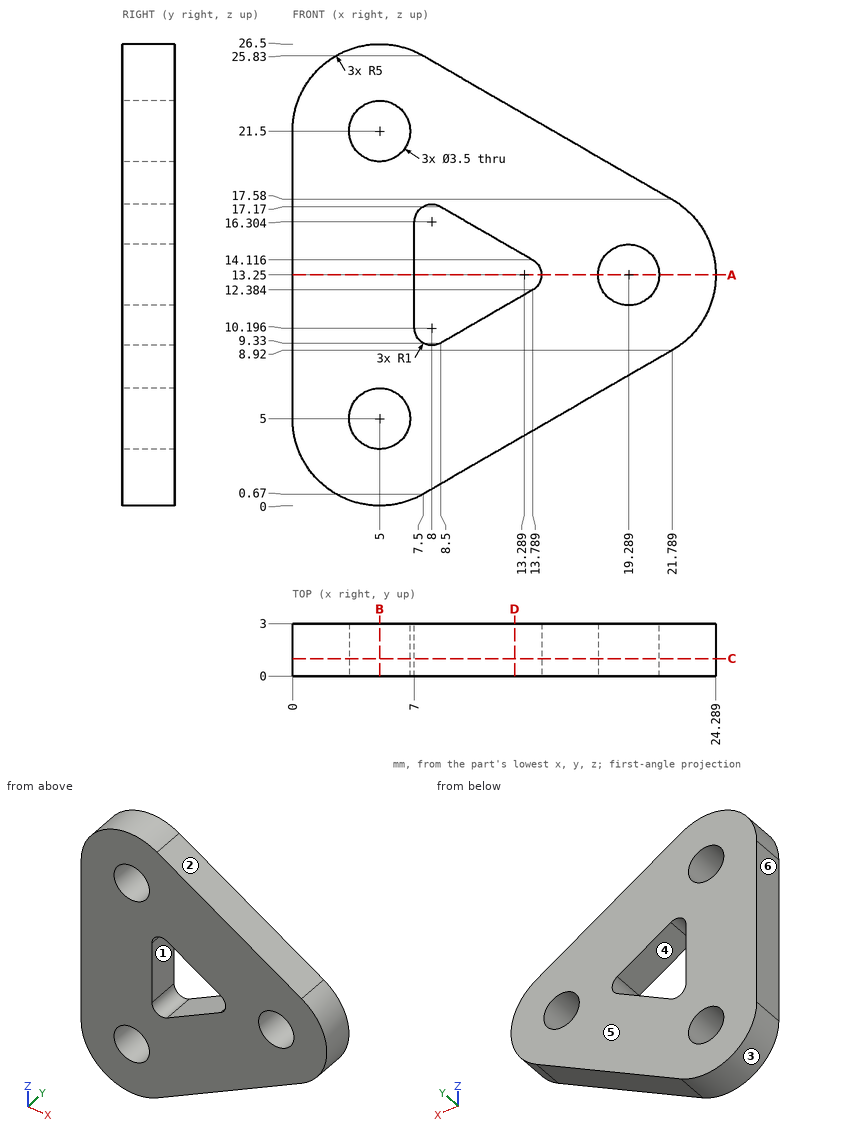
Part print with two shaded views. Sizes in mm from the minimum x, y, z corner. A direction names the side the tool comes from. Give positions to 0.01 mm unless a question says otherwise; leave off trailing zeros. Order: outer loops, then holes, each group sorted by start corner. A loop starts at its lowest first (then second) coordinate and runs counter-clockwise, first axis right, second up.
(1) Saw through at A-A, the plane z = 13.25. Give the cut face in (x, y).
(2) Drill centre lines: L1, parallel to Z at x = 5, y = 0.65; L2, parallel to X at y = 2.15, z = 14.75 (1 decimal); L3, parallel to X at y = 1.65, z = 12 (1 decimal). Where is each one in solid material? Low to high.
(3) Tool access for the marked faces 1 and 2: list every direction of +Z, -Z, +X, -X, +Y, -Y with a clear straight run to the whole face (end or side of a thin tool).
(4) Saw through at B-B, the plane x = 5. Give the cut face in (y, z).
(5) Saw through at C-C, the plane y = 1. Give the cut face in (x, z).
(6) Saw through at D-D, the plane x = 12.75. Give the cut face in (y, z).
(7) Mould opens along X. For the marked faces 3, 4, 5 and 6 say: released by +X, released by -X, zero draft, split by the parting line, or undercut.
(8) Flat gauge pins, fed straight in: pin 1 (1.5 mm diameter, centred on x = 9, y = 1.5, fed in from +Z); pin 2 (1.5 mm diameter, centred on y = 0.5, z = 3.5, fed in from -X). Where does each tip first touch, or does it go through?
Results found:
1. outline: (0, 0) - (7, 0) - (7, 3) - (0, 3) - close; (14.29, 0) - (17.54, 0) - (17.54, 3) - (14.29, 3) - close; (21.04, 0) - (24.29, 0) - (24.29, 3) - (21.04, 3) - close
2. L1: z = 0 to 3.25, 6.75 to 19.75, 23.25 to 26.5
2. L2: x = 0 to 7, 12.7 to 18.4, 20.2 to 24.1
2. L3: x = 0 to 7, 13.1 to 18.1, 20.5 to 24.1
3. face 1: +Y, -Y
3. face 2: +Z, +X, +Y, -Y
4. outline: (0, 0) - (3, 0) - (3, 3.25) - (0, 3.25) - close; (0, 6.75) - (3, 6.75) - (3, 19.75) - (0, 19.75) - close; (0, 23.25) - (3, 23.25) - (3, 26.5) - (0, 26.5) - close
5. outline: (0, 5) arc R5 ccw to (7.5, 0.67) - (21.79, 8.92) arc R5 ccw to (21.79, 17.58) - (7.5, 25.83) arc R5 ccw to (0, 21.5) - close; hole circle Ø3.5 at (5, 5); hole circle Ø3.5 at (5, 21.5); hole (7, 10.2) arc R1 ccw to (8.5, 9.33) - (13.79, 12.38) arc R1 ccw to (13.79, 14.12) - (8.5, 17.17) arc R1 ccw to (7, 16.3) - close; hole circle Ø3.5 at (19.29, 13.25)
6. outline: (0, 3.7) - (3, 3.7) - (3, 11.78) - (0, 11.78) - close; (0, 14.72) - (3, 14.72) - (3, 22.8) - (0, 22.8) - close
7. face 3: split by the parting line
7. face 4: undercut
7. face 5: zero draft
7. face 6: released by -X
8. pin 1: stops at z = 25.4
8. pin 2: stops at x = 0.06
